The model under review builds one solid part; all positions refer to its coordinate system, in mm. A direction names the side the tool comes from. Give positions to 0.01 mm unless a question says otherwise; leave off trailing zeros. Loops run counter-clockwise (first coordinate to the right, second up) from the corner with the lowest first, then second, coordinate; pieces in that order, holes last. Notation, with made-up numbers: (-2, 83) - (52, 83) arc R27 ccw to (52, 121) - close; hole circle Ø6 at (63.25, -1). An arc over 180 degrees is marked (long way). Return JSON: item names as keys, results as strings. Group by question number.
from build123d import *

# Parameters (mm, degrees)
BOSS_EXTRUDE2_DEPTH = 2.5
SKETCH3_W           = 10
SKETCH3_H           = 14.5
CUT_EXTRUDE3_DEPTH  = 40


with BuildPart() as part:
    # Sketch1 → Boss-Extrude2 (new body)
    with BuildSketch(Plane(origin=(0, 0, 0), x_dir=(1, 0, 0), z_dir=(0, 1, 0))):
        with BuildLine():
            Line((-52.5, 32.5), (-41.25, 32.5))
            Line((-41.25, 32.5), (-41.25, 35))
            Line((-41.25, 35), (-11.25, 35))
            Line((-11.25, 35), (-11.25, 32.5))
            Line((-11.25, 32.5), (11.25, 32.5))
            Line((11.25, 32.5), (11.25, 35))
            Line((11.25, 35), (41.25, 35))
            Line((41.25, 35), (41.25, 32.5))
            Line((41.25, 32.5), (52.5, 32.5))
            ThreePointArc((52.5, 32.5), (66.642135624, 26.642135624), (72.5, 12.5))
            Line((72.5, 12.5), (72.5, -12.5))
            ThreePointArc((72.5, -12.5), (66.642135624, -26.642135624), (52.5, -32.5))
            Line((52.5, -32.5), (41.25, -32.5))
            Line((41.25, -32.5), (41.25, -35))
            Line((41.25, -35), (11.25, -35))
            Line((11.25, -35), (11.25, -32.5))
            Line((11.25, -32.5), (-11.25, -32.5))
            Line((-11.25, -32.5), (-11.25, -35))
            Line((-11.25, -35), (-41.25, -35))
            Line((-41.25, -35), (-41.25, -32.5))
            Line((-41.25, -32.5), (-52.5, -32.5))
            ThreePointArc((-52.5, -32.5), (-66.642135624, -26.642135624), (-72.5, -12.5))
            Line((-72.5, -12.5), (-72.5, 12.5))
            ThreePointArc((-72.5, 12.5), (-66.642135624, 26.642135624), (-52.5, 32.5))
        make_face()
    extrude(amount=BOSS_EXTRUDE2_DEPTH)

    # Sketch3 → Cut-Extrude3 (cut)
    with BuildSketch(Plane.XZ):
        Rectangle(SKETCH3_W, SKETCH3_H)
    extrude(amount=-CUT_EXTRUDE3_DEPTH, mode=Mode.SUBTRACT)


solid = part.part
Item 1: Take a section at A-A (z = -3). State the section outline as (x, y) points, then the cut area to 4 significant figures.
Item 2: For L1, parallel to X at y = 0.4, z = 5; L2, parallel to Z at x = 9, y = 0.9; L3, parallel to X at y = 0.55, z = -22, list the stretches that pass through material, from the lowest coordinate up. Write a range as from..to.
Item 3: For P1, Ø0.8, axis at x = 48, y = 1, coming from the +Z side; P2, Ø0.8, axis at y = 1.5, z = -34.5, coming from the +X side; P3, Ø0.8, axis at y = 0.5, z = 33.5, coming from the -X side, all flat-tipped, find the tip position at first contact; note any pin that passes through.
Item 4: Take a section at D-D (z = -27). State the section outline as (x, y) points.
Item 5: Tool access review of faces 4 (the face through (47, 1, -32.5)), 5 (the face through (-11.25, 1, 34)), 6 (the face through (-41.25, 1, 34)): name each direction out of +Z, -Z, +X, -X, +Y, -Y from which nothing blocks a thin tool from reaching the whole face with its end or side.
Item 6: Mouldability with a two-part tool opening along Z and no side actions: class faces 1 (the face through (-66.797, 1.232, -26.486)), 2 (the face through (-72.5, 1, 0)), 3 (the face through (5, 1, 0)) as +Z half, -Z half, draft (parallel to the pull), parting line (faces both ways), or undercut.
Item 7: Take a section at C-C (x = -62). State the section outline as (y, z) points.
Item 8: Take a section at B-B (y = 0.4). State the section outline as (x, z) points.
Check sheet entries:
{
 "1": {"outline": "(-72.5, 0) - (-5, 0) - (-5, 2.5) - (-72.5, 2.5) - close; (5, 0) - (72.5, 0) - (72.5, 2.5) - (5, 2.5) - close", "area": "337.5 mm^2"},
 "2": {"L1": "x = -72.5..-5, 5..72.5", "L2": "z = -32.5..32.5", "L3": "x = -70.1..70.1"},
 "3": {"P1": "stops at z = 32.5", "P2": "stops at x = 41.25", "P3": "stops at x = -41.25"},
 "4": {"outline": "(-66.27, 0) - (66.27, 0) - (66.27, 2.5) - (-66.27, 2.5) - close"},
 "5": {"face 4": "-Z, +X, +Y, -Y", "face 5": "+Z, +Y, -Y", "face 6": "+Z, -X, +Y, -Y"},
 "6": {"face 1": "-Z half", "face 2": "draft", "face 3": "undercut"},
 "7": {"outline": "(0, -30.1) - (2.5, -30.1) - (2.5, 30.1) - (0, 30.1) - close"},
 "8": {"outline": "(-72.5, -12.5) arc R20 ccw to (-52.5, -32.5) - (-41.25, -32.5) - (-41.25, -35) - (-11.25, -35) - (-11.25, -32.5) - (11.25, -32.5) - (11.25, -35) - (41.25, -35) - (41.25, -32.5) - (52.5, -32.5) arc R20 ccw to (72.5, -12.5) - (72.5, 12.5) arc R20 ccw to (52.5, 32.5) - (41.25, 32.5) - (41.25, 35) - (11.25, 35) - (11.25, 32.5) - (-11.25, 32.5) - (-11.25, 35) - (-41.25, 35) - (-41.25, 32.5) - (-52.5, 32.5) arc R20 ccw to (-72.5, 12.5) - close; hole (-5, -7.25) - (5, -7.25) - (5, 7.25) - (-5, 7.25) - close"}
}
